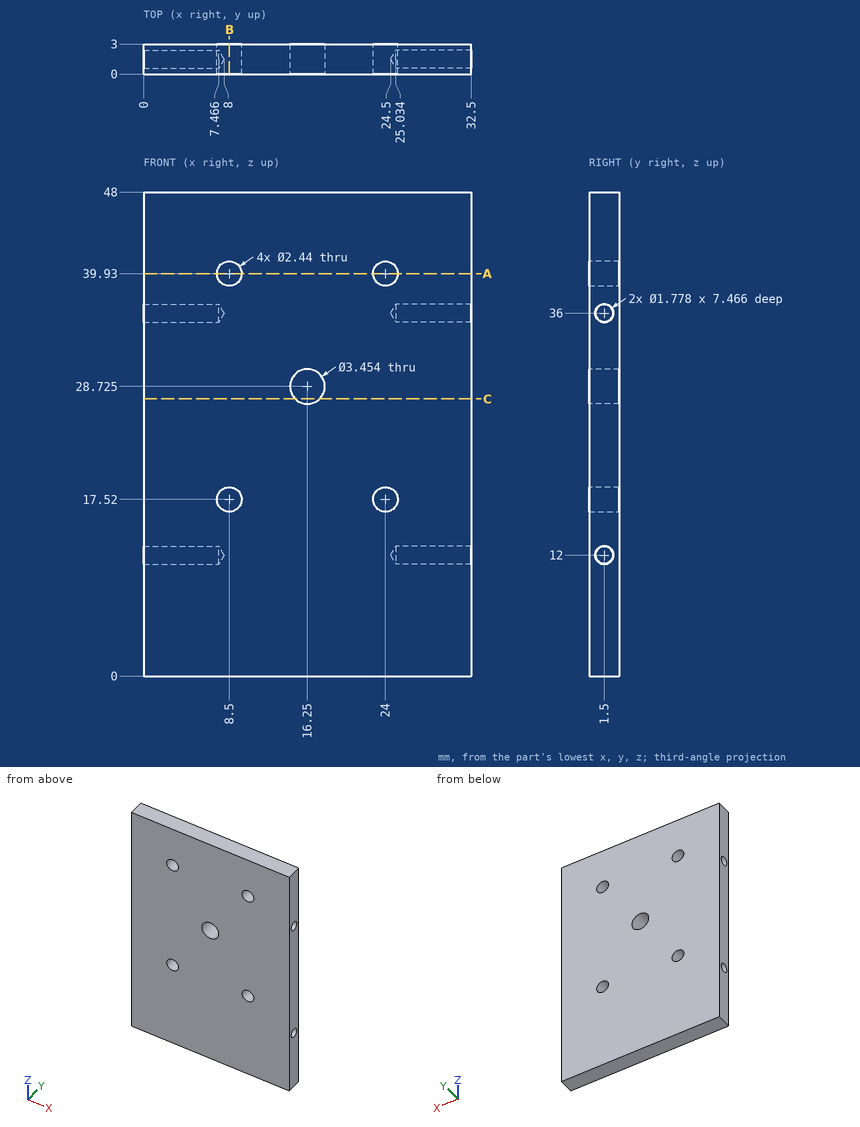
Drawing for the job (mm, zero at the part's lowest x, y, z). Round coordinates to 2 decimals unless told otherwise and drop trailing zeros. Loops run counter-clockwise (first coordinate to the right, second up) from the corner with the lowest first, then second, coordinate; pieces in that order, holes last. Notation, with made-up numbers: (69.5, -26.5) -> (74.5, -26.5) arc R5 cw to (74.5, -22.5) -> close; hole circle Ø7 at (-3.75, 43.25). An arc over 180 degrees is marked (long way). Use one line per item in the form item = value. Start each with the question number.
Item 1: Band-saw the part on C-C (z = 27.5). List the corners of the cut face in (x, y).
Item 2: Drop flat-ended pins along their axis: pin 1 Ø3 at (x, z) = (24, 17.52) entering from -Y; pin 2 Ø1.1 at (y, z) = (1.5, 12) entering from +X. Give the stop position or say it passes through.
Item 3: Drill centre lines: line 1 along X through (y, z) = (2.25, 39.93); line 2 along Z through (x, y) = (4.25, 1.5); line 3 along Y through (x, z) = (5, 36). Where is each one in solid material? Low to high.
Item 4: Band-saw the part on A-A (z = 39.93). List the corners of the cut face in (x, y).
Item 5: Band-saw the part on B-B (x = 8.5). List the corners of the cut face in (y, z).
Data:
q1.outline = (0, 0) -> (15.03, 0) -> (15.03, 3) -> (0, 3) -> close; (17.47, 0) -> (32.5, 0) -> (32.5, 3) -> (17.47, 3) -> close
q2.pin_1 = 0
q2.pin_2 = 24.83
q3.line_1 = 0 to 7.28, 9.72 to 22.78, 25.22 to 32.5
q3.line_2 = 0 to 11.11, 12.89 to 35.11, 36.89 to 48
q3.line_3 = 0 to 0.61, 2.39 to 3
q4.outline = (0, 0) -> (7.28, 0) -> (7.28, 3) -> (0, 3) -> close; (9.72, 0) -> (22.78, 0) -> (22.78, 3) -> (9.72, 3) -> close; (25.22, 0) -> (32.5, 0) -> (32.5, 3) -> (25.22, 3) -> close
q5.outline = (0, 0) -> (3, 0) -> (3, 16.3) -> (0, 16.3) -> close; (0, 18.74) -> (3, 18.74) -> (3, 38.71) -> (0, 38.71) -> close; (0, 41.15) -> (3, 41.15) -> (3, 48) -> (0, 48) -> close
